For this review, use the dimensioned drawing (mm, ordinates from the lowest corner) and the shaded views. A direction names the side the tool comes from. Coordinates: 2 decimals unless noted, no trailing zeros. Loops run counter-clockwise (first coordinate to the right, second up) from the corner with the lowest first, then second, coordinate; pieces in that order, holes last. Notation, with made-up numbers: M 59.25,-17 L 110.25,-17 A15 cw 110.25,-12 Z; hole C -29,26.5 d7. An arc over 180 degrees is marked long. Write item = value, one per line.
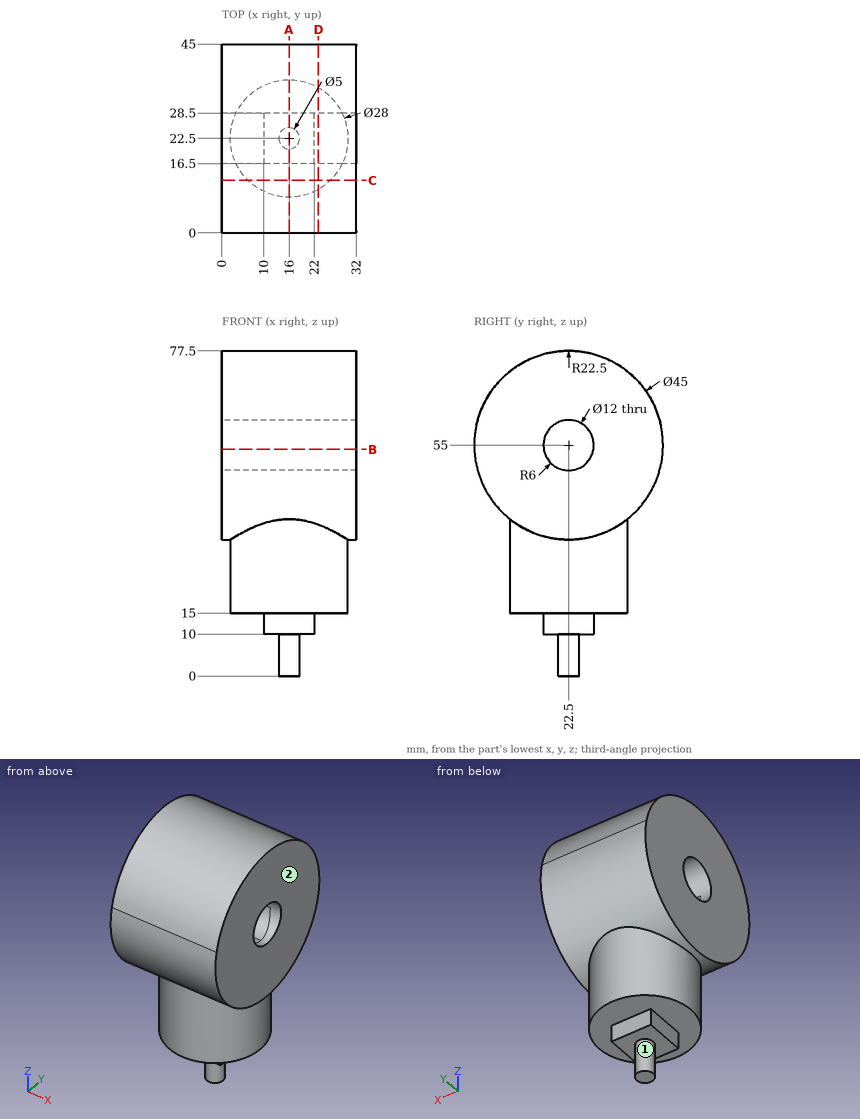
Q1. For pin 1 Ø1.5 at (y, z) = (20.5, 11.5) entering from +X; pin 2 Ø4 at (x, z) = (22, 64.5) entering from -Y; pin 3 Ø1 at (y, z) = (29.5, 12) entering from +X; pin 4 Ø8 at (y, z) = (11, 21.5) entering from -X, all flat-tipped, find the tip position at first contact; note any pin that passes through.
Solved:
pin_1 = 22
pin_2 = 1.29
pin_3 = through
pin_4 = 4.18
Q2. Add section B-B (z = 54). Write out the cut boundary in (x, y).
Solved:
outline = M 0,0.02 L 32,0.02 L 32,16.58 L 0,16.58 Z; M 0,28.42 L 32,28.42 L 32,44.98 L 0,44.98 Z
Q3. For line 1 along Y through (x, z) = (13, 55); line 2 along Z through (x, y) = (8.5, 26.5); line 3 along Y through (x, z) = (1, 52), list the stretches that pass through material, from the lowest coordinate up.
Solved:
line_1 = 0 to 16.5, 28.5 to 45
line_2 = 15 to 50.53, 59.47 to 77.14
line_3 = 0.2 to 17.3, 27.7 to 44.8
Q4. Add section C-C (y = 12.5). Write out the cut boundary in (x, z).
Solved:
outline = M 0,34.84 L 6.2,34.84 L 6.2,15 L 25.8,15 L 25.8,34.84 L 32,34.84 L 32,75.16 L 0,75.16 Z
Q5. Add section D-D (x = 23). Write out the cut boundary in (y, z), and give its area (3 significant figures).
Solved:
outline = M 10.38,15 L 34.62,15 L 34.62,36.05 A22.5 ccw long 10.38,36.05 Z; hole C 22.5,55 d12
area = 1,930 mm²
Q6. Machinability: for the marked faces 1 and 2, which of the approach directions +Z, -Z, +X, -X, +Y, -Y give a long, thin tool a straight path to every point of the face, cutting with its end or side? Answer none if there is none.
Solved:
face_1 = -Z
face_2 = +Z, -Z, +X, +Y, -Y
Q7. Add section A-A (x = 16). Write out the cut boundary in (y, z).
Solved:
outline = M 8.5,15 L 16.5,15 L 16.5,10 L 20,10 L 20,0 L 25,0 L 25,10 L 28.5,10 L 28.5,15 L 36.5,15 L 36.5,37.39 A22.5 ccw long 8.5,37.39 Z; hole C 22.5,55 d12
